Geometry: see drawing. Coordinates: mm, zero at the bounding-box minimum. Round coordinates to 2 decimals unless told otherwise and drop trailing zeros. Order: outer loops, then holes, each group sorted by start corner. A loop starts at its lowest first (then second) coordinate and runs counter-clockwise, first axis right, second up. Notation, with made-up numbers: (3.25, 70.5) -> (55.25, 70.5) arc R20 ccw to (55.25, 93.5) -> close; hole circle Ø2 at (63, -7.75). An arc over 180 degrees is marked (long way). Use a Markdown table: item, result.
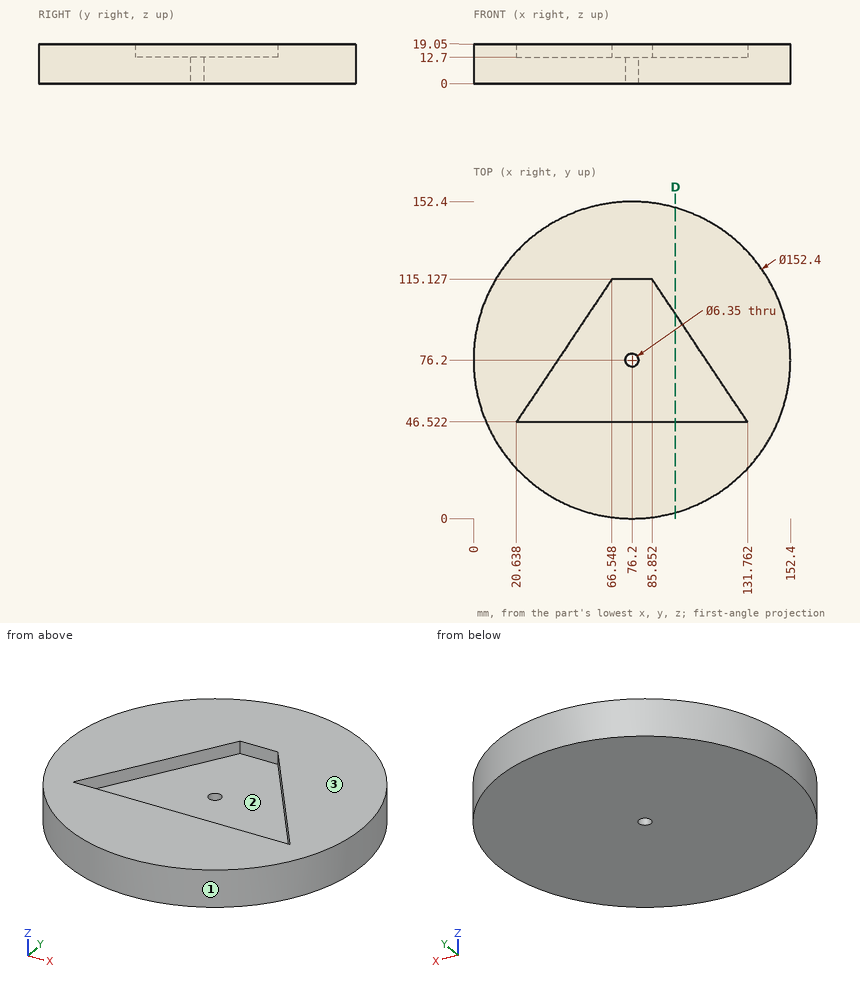
1) Cut plane D-D on x = 97. Return loops of the section in (y, z).
Answer key:
| item | result |
|---|---|
| outline | (2.89, 0) -> (149.51, 0) -> (149.51, 19.05) -> (98.47, 19.05) -> (98.47, 12.7) -> (46.52, 12.7) -> (46.52, 19.05) -> (2.89, 19.05) -> close |
2) Contact query for flat-ended pins moving along their axis: P1, Ø1, axis at x = 59, z = 7, coming from the +Y side; P2, Ø7, axis at x = 103.5, z = 17, coming from the +Y side; P3, Ø1, axis at x = 25.5, z = 12.5, coming from the -Y side. Output: stop coordinate, or through.
Answer key:
| item | result |
|---|---|
| P1 | stops at y = 150.55 |
| P2 | stops at y = 148.59 |
| P3 | stops at y = 18.87 |
3) Draft query along X for the marked faces 1, 2 and 3. Return one class per face: released by +X, released by -X, zero draft, split by the parting line, or undercut.
Answer key:
| item | result |
|---|---|
| face 1 | split by the parting line |
| face 2 | undercut |
| face 3 | zero draft |
4) Ray query, probe 1 along Y at (x, z) = (76.2, 2.5) (1 decimal); probe 2 along Z at (x, y) = (78.5, 103.5); probe 3 along Y at (x, z) = (96, 15.5) (1 decimal). Return the intervals inside material, ascending.
Answer key:
| item | result |
|---|---|
| probe 1 | y = 0 to 73, 79.4 to 152.4 |
| probe 2 | z = 0 to 12.7 |
| probe 3 | y = 2.6 to 46.5, 100 to 149.8 |
